from build123d import *

# Parameters (mm, degrees)
F0_W       = 1
F0_H       = 1
F1_DEPTH   = 7
F2_SIZE2   = 2.747467
F2_SIZE    = 0.99999
F2_2_SIZE2 = 2.747467
F2_2_SIZE  = 0.99999
F3_SIZE2   = 2.904201
F3_SIZE    = 0.99999


# Not quite as in the source:
# - a fillet or chamfer is up to 0.001 mm smaller than in the source, because OpenCascade refuses the exact size


with BuildPart() as f1:
    # F0 (on Front) → F1 (new body)
    with BuildSketch(Plane.XZ):
        Polygon((-56.745035848, 28.2884484402), (-56.745035848, 26.7884484402), (-56.745035848, 25.2884484402), (-51.245035848, 25.2884484402), (-51.245035848, 26.2884484402), (-51.745035848, 26.2884484402), (-51.745035848, 27.2884484402), (-51.245035848, 27.2884484402), (-51.245035848, 28.2884484402), (-52.245035848, 28.2884484402), (-53.245035848, 28.2884484402), (-54.245035848, 28.2884484402), align=None)
        Polygon((-54.745035848, 26.2884484402), (-55.745035848, 26.2884484402), (-55.745035848, 26.7884484402), (-55.745035848, 27.2884484402), (-54.745035848, 27.2884484402), align=None, mode=Mode.SUBTRACT)
        with Locations((-53.245035848, 26.7884484402)):
            Rectangle(F0_W, F0_H, mode=Mode.SUBTRACT)
        Polygon((-50.745035848, 26.7884484402), (-49.745035848, 26.7884484402), (-49.745035848, 28.2884484402), (-51.245035848, 28.2884484402), (-51.245035848, 27.2884484402), (-50.745035848, 27.2884484402), align=None)
        Polygon((-51.245035848, 26.2884484402), (-51.245035848, 25.2884484402), (-49.745035848, 25.2884484402), (-49.745035848, 26.7884484402), (-50.745035848, 26.7884484402), (-50.745035848, 26.2884484402), align=None)
        with Locations((-52.745035848, 28.7884484402)):
            Rectangle(F0_W, F0_H)
        with Locations((-53.745035848, 28.7884484402)):
            Rectangle(F0_W, F0_H)
    extrude(amount=F1_DEPTH)

    # F2 (size 1 and 2.7474774195 in the source; OpenCascade refuses exactly that, so slightly less here)
    f2_edges = [f1.edges().sort_by_distance(p)[0] for p in [
        (-51.245036, 0, 26.288448),
        (-51.245036, 0, 27.288448),
        (-53.245036, 0, 27.288448),
        (-53.245036, 0, 26.288448),
        (-55.245036, 0, 27.288448),
        (-55.245036, 0, 26.288448),
    ]]
    f2_side = f1.faces().sort_by_distance((-56.664413, 0, 26.788448))[0]
    chamfer(f2_edges, length=F2_SIZE, length2=F2_SIZE2, reference=f2_side)

    # F2#2 (size 1 and 2.7474774195 in the source; OpenCascade refuses exactly that, so slightly less here)
    f2_2_edges = [f1.edges().sort_by_distance(p)[0] for p in [
        (-55.245036, -7, 27.288448),
        (-53.245036, -7, 27.288448),
        (-51.245036, -7, 27.288448),
    ]]
    f2_2_side = f1.faces().sort_by_distance((-56.664413, -7, 26.788448))[0]
    chamfer(f2_2_edges, length=F2_2_SIZE, length2=F2_2_SIZE2, reference=f2_2_side)

    # F3 (size 1 and 2.9042108777 in the source; OpenCascade refuses exactly that, so slightly less here)
    f3_edges = [f1.edges().sort_by_distance(p)[0] for p in [
        (-55.245036, -7, 26.288448),
        (-53.245036, -7, 26.288448),
        (-51.245036, -7, 26.288448),
    ]]
    f3_side = f1.faces().sort_by_distance((-55.825658, -7, 27.788443))[0]
    chamfer(f3_edges, length=F3_SIZE, length2=F3_SIZE2, reference=f3_side)


solid = f1.part
Model file for the job. Use its own axes, mm. A direction names the side the tool comes from. Give positions to 0.01 mm unless a question says otherwise; leave off trailing zeros. Loops run counter-clockwise (first coordinate to the right, second up) from the corner with the lowest first, then second, coordinate; pieces in that order, holes last. Notation, with made-up numbers: (-6, 70) -> (6, 70) arc R23 ccw to (6, 88) -> close; hole circle Ø2 at (-5, 64.25). An arc over 180 degrees is marked (long way). Use a Markdown table: item, result. Add a question column.
(1) Slice it at A-A on z = 26.7. List the corners of the cut face in (x, y), and give its area (3 significant figures).
(2) Tool access for faces 4 (the flat face through (-53.3, -1.4, 25.8)), 5 (the flat face through (-51.238, -5.528, 25.795)), 6 (the flat face through (-55.745, -3, 27)): list every direction of +Z, -Z, +X, -X, +Y, -Y with a clear straight run to the whole face (end or side of a thin tool).
(3) Slice it at D-D on z = 28.7. List the corners of the cut face in (x, y), and give its area (3 significant figures).
(4) Mould opens along Z. For faces 1 (the flat face through (-53.252, -5.528, 25.795)), 2 (the flat face through (-53, -3, 25.288)), 3 (the flat face through (-56.745, -3, 27)) say: +Z half, -Z half, draft (parallel to the pull), parting line (faces both ways), or undercut.
(5) Wall check: line 1 along X through (y, z) = (-6.25, 26.5); line 2 along Z through (x, y) = (-53, -3.25); line 3 along Z through (x, y) = (-55.5, -5.25). Give the ranges that are in metal, low to high.
(6) Drop flat-ended pins along their axis: pin 1 Ø1 at (x, z) = (-55, 28) entering from -Y; pin 2 Ø0.5 at (x, y) = (-55, -3) entering from +Z. Give the stop position or say it passes through.
(7) Slice it at C-C on y = -1.75. List the corners of the cut face in (x, z), and give its area (3 significant figures).
Filled sheet:
| question | item | result |
|---|---|---|
| 1 | outline | (-56.75, -7) -> (-55.75, -7) -> (-55.75, 0) -> (-56.75, 0) -> close; (-54.75, -7) -> (-53.75, -7) -> (-53.75, 0) -> (-54.75, 0) -> close; (-52.75, -7) -> (-51.75, -7) -> (-51.75, 0) -> (-52.75, 0) -> close; (-50.75, -7) -> (-49.75, -7) -> (-49.75, 0) -> (-50.75, 0) -> close |
| 1 | area | 28.0 mm2 |
| 2 | face 4 | +Y |
| 2 | face 5 | -Y |
| 2 | face 6 | none |
| 3 | outline | (-54.25, -7) -> (-52.25, -7) -> (-52.25, 0) -> (-54.25, 0) -> close |
| 3 | area | 14.0 mm2 |
| 4 | face 1 | undercut |
| 4 | face 2 | -Z half |
| 4 | face 3 | draft |
| 5 | line 1 | -56.75 to -55.75, -54.75 to -53.75, -52.75 to -51.75, -50.75 to -49.75 |
| 5 | line 2 | 25.29 to 26.29, 27.29 to 29.29 |
| 5 | line 3 | 25.29 to 25.89, 27.65 to 28.29 |
| 6 | pin 1 | y = -7 |
| 6 | pin 2 | z = 28.29 |
| 7 | outline | (-56.75, 25.29) -> (-49.75, 25.29) -> (-49.75, 28.29) -> (-52.25, 28.29) -> (-52.25, 29.29) -> (-54.25, 29.29) -> (-54.25, 28.29) -> (-56.75, 28.29) -> close; hole (-55.75, 25.93) -> (-54.75, 25.93) -> (-54.75, 27.65) -> (-55.75, 27.65) -> close; hole (-53.75, 25.93) -> (-52.75, 25.93) -> (-52.75, 27.65) -> (-53.75, 27.65) -> close; hole (-51.75, 25.93) -> (-50.75, 25.93) -> (-50.75, 27.65) -> (-51.75, 27.65) -> close |
| 7 | area | 17.8 mm2 |
